```python
from build123d import *

# Parameters (mm, degrees)
F1_DEPTH = 1.1
F2_W     = 9.1
F2_H     = 8.9
F2_W_2   = 8.9
F2_H_2   = 9.1
F3_DEPTH = 6.1
F2_R     = 1
F4_DEPTH = 1.101


with BuildPart() as f1:
    # F0 (on Top) → F1 (new body)
    with BuildSketch(Plane.XY):
        Polygon((-11.5, 11.5), (-23, 11.5), (-23, 0), (-11.5, 0), (-11.5, -12), (0, -12), (0, 0), (11.5, 0), (11.5, 11.5), (0, 11.5), (0, 23.5), (-11.5, 23.5), align=None)
    extrude(amount=F1_DEPTH)

    # F2 (on face) → F3 (join)
    with BuildSketch(Plane.XY.offset(1.1)):
        with Locations((-17.15, 5.75)):
            Rectangle(F2_W, F2_H)
        Polygon((-8.575388, 5.75), (-12.6, 10.2), (-12.6, 1.3), align=None)
        Polygon((-5.75, 2.924612), (-10.2, -1.1), (-1.3, -1.1), align=None)
        with Locations((-5.75, -5.65)):
            Rectangle(F2_W_2, F2_H_2)
        with Locations((5.65, 5.75)):
            Rectangle(F2_W, F2_H)
        Polygon((1.1, 1.3), (1.1, 10.2), (-2.924612, 5.75), align=None)
        Polygon((-1.3, 12.6), (-10.2, 12.6), (-5.75, 8.575388), align=None)
        with Locations((-5.75, 17.15)):
            Rectangle(F2_W_2, F2_H_2)
    extrude(amount=F3_DEPTH)

    # F2 (on face) → F4 (cut, through all)
    with BuildSketch(Plane.XY.offset(1.1)):
        with Locations((-5.75, 5.249888)):
            Circle(F2_R)
    extrude(amount=-F4_DEPTH, mode=Mode.SUBTRACT)


solid = f1.part
```
Here's how the part is built. I have some questions about the finished solid (model axes, mm). A direction names the side the tool comes from. Round coordinates to 2 decimals unless told otherwise and drop trailing zeros. Order: outer loops, then holes, each group sorted by start corner. A loop starts at its lowest first (then second) coordinate and runs counter-clockwise, first axis right, second up. Notation, with made-up numbers: M 69.5,10 L 86.5,10 A11 ccw 86.5,15 Z; hole C 49.5,55.5 d3. An arc over 180 degrees is marked long. Answer as CSV lines item,"result".
Item 1: We'd pull the mould along X, two halves only. Please class faces 1 (the flat face through (0, 17.4, 0.5)), 2 (the flat face through (5.8, 11.5, 0.5)), 3 (the flat face through (-7.944, 0.94, 4.107)): +X half, -X half, draft (parallel to the pull), parting line (faces both ways), or undercut.
From the geometry:
face 1,"+X half"
face 2,"draft"
face 3,"undercut"
Item 2: Please list where these lines run through material, in increasing order: L1, parallel to Y at x = -5.75, z = 0.85; L2, parallel to X at y = 2.5, z = 1.5; L3, parallel to Y at x = -2, z = 2.75. Write a range as [from, to].
From the geometry:
L1,"[-12, 4.25], [6.25, 23.5]"
L2,"[-21.7, -11.51], [-6.22, -5.28], [0.01, 10.2]"
L3,"[-10.2, -0.47], [4.73, 6.77], [11.97, 21.7]"
Item 3: Imagine slicing it at B-B on x = -19.5. List the corners of the cut face in (y, z) for me.
From the geometry:
outline,"M 0,0 L 11.5,0 L 11.5,1.1 L 10.2,1.1 L 10.2,7.2 L 1.3,7.2 L 1.3,1.1 L 0,1.1 Z"
Item 4: Imagine slicing it at A-A on z = 3.5. List the corners of the cut face in (x, y) for me, and give its area (3 significant figures).
From the geometry:
outline,"M -21.7,1.3 L -12.6,1.3 L -8.58,5.75 L -12.6,10.2 L -21.7,10.2 Z; M -10.2,-10.2 L -1.3,-10.2 L -1.3,-1.1 L -5.75,2.92 L -10.2,-1.1 Z; M -10.2,12.6 L -5.75,8.58 L -1.3,12.6 L -1.3,21.7 L -10.2,21.7 Z; M -2.92,5.75 L 1.1,1.3 L 10.2,1.3 L 10.2,10.2 L 1.1,10.2 Z"
area,"396 mm2"
Item 5: Imagine slicing it at C-C on x = -2.5. List the corners of the cut face in (y, z) for me, and give its area (3 significant figures).
From the geometry:
outline,"M -12,0 L 23.5,0 L 23.5,1.1 L 21.7,1.1 L 21.7,7.2 L 11.51,7.2 L 11.51,1.1 L 6.22,1.1 L 6.22,7.2 L 5.28,7.2 L 5.28,1.1 L -0.01,1.1 L -0.01,7.2 L -10.2,7.2 L -10.2,1.1 L -12,1.1 Z"
area,"169 mm2"
Item 6: Which directions (+Z, -Z, +X, -X, +Y, -Y) give clear straight access to the entire face, cutting with the end or side of a thin tool? Please do faces 4 (the flat face through (-17.3, 0, 0.5)), 5 (the flat face through (10.2, 6, 4)), 6 (the flat face through (-10.56, 7.944, 4.107)), 7 (the flat face through (6, 10.2, 4)), 8 (the flat face through (-6, -10.2, 4)).
From the geometry:
face 4,"+Z, -Z, -X, -Y"
face 5,"+Z, +X, +Y, -Y"
face 6,"+Z"
face 7,"+Z, +X, +Y"
face 8,"+Z, +X, -X, -Y"
Item 7: For pin 1 (3 mm diameter, centred on x = 3.5, z = 3.5, fed in from -Y); pin 2 (1.8 mm diameter, centred on y = -4, z = 4.5, fed in from -X); pin 3 (1.8 mm diameter, centred on x = -18, z = 5.5, fed in from +Y); pin 4 (12 mm diameter, centred on x = -11, y = 12.5, fed in from +Z), each with a flat end and sliding along its axis, tell me the tip position at first contact or that it passes through.
From the geometry:
pin 1,"y = 1.3"
pin 2,"x = -10.2"
pin 3,"y = 10.2"
pin 4,"z = 7.2"
